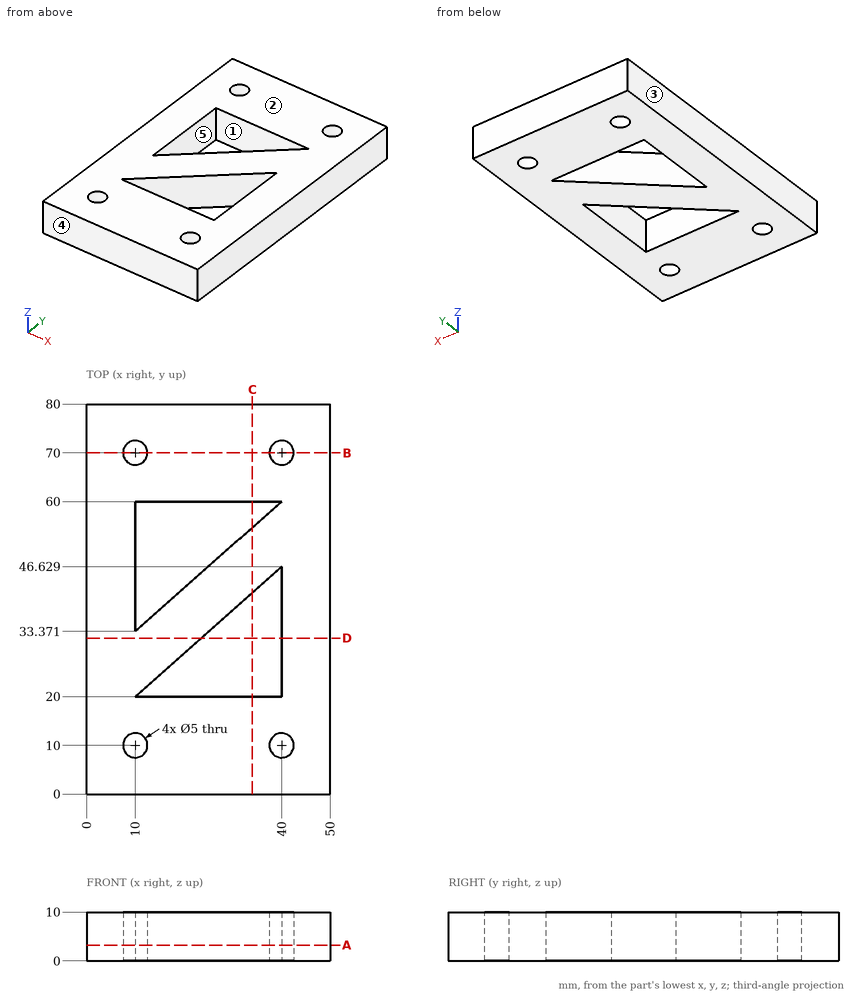
Geometry: see drawing. Coordinates: mm, zero at the bounding-box minimum. A direction names the side the tool comes from. Give positions to 0.01 mm unless a question says otherwise; leave off trailing zeros. Order: outer loops, then holes, each group sorted by start corner. A loop starts at its lowest first (then second) coordinate and runs counter-clockwise, first axis right, second up.
Q1. Section D-D on y = 32. Output: boundary loops of the cut face in (x, z), and give its area (3 significant figures).
Checked values:
outline: (0, 0) - (23.52, 0) - (23.52, 10) - (0, 10) - close; (40, 0) - (50, 0) - (50, 10) - (40, 10) - close
area: 335 mm2
Q2. Ray query, probe 1 along Y at (x, z) = (24, 8.5); probe 2 along Y at (x, z) = (33, 2.25) (1 decimal); probe 3 along X at (y, z) = (69.5, 8.75). Return the intervals inside material, ascending.
Checked values:
probe 1: y = 0 to 20, 32.43 to 45.8, 60 to 80
probe 2: y = 0 to 20, 40.4 to 53.8, 60 to 80
probe 3: x = 0 to 7.55, 12.45 to 37.55, 42.45 to 50
Q3. Contact query for a flat-ended pin moving along its axis: pin 1 Ø4 at (x, y) = (10, 10) entering from -Z. Output: stop coordinate, or through.
Checked values:
pin 1: passes through
Q4. Section B-B on y = 70. Output: boundary loops of the cut face in (x, z).
Checked values:
outline: (0, 0) - (7.5, 0) - (7.5, 10) - (0, 10) - close; (12.5, 0) - (37.5, 0) - (37.5, 10) - (12.5, 10) - close; (42.5, 0) - (50, 0) - (50, 10) - (42.5, 10) - close
Q5. Section C-C on x = 34. Output: boundary loops of the cut face in (y, z).
Checked values:
outline: (0, 0) - (20, 0) - (20, 10) - (0, 10) - close; (41.3, 0) - (54.67, 0) - (54.67, 10) - (41.3, 10) - close; (60, 0) - (80, 0) - (80, 10) - (60, 10) - close
Q6. Set-up query: the marked faces 1 and 2. Return all of +Z, -Z, +X, -X, +Y, -Y with unobstructed straight access to the full face (end or side cutting, diameter ignored); none if empty.
Checked values:
face 1: +Z, -Z
face 2: +Z, +X, -X, +Y, -Y
Q7. Draft query along Y for the marked faces 3, 4 and 5. Return one class per face: +Y half, -Y half, draft (parallel to the pull), parting line (faces both ways), or undercut.
Checked values:
face 3: draft
face 4: -Y half
face 5: undercut
Q8. Section A-A on z = 3.25. Output: boundary loops of the cut face in (x, y), and give its area (3 significant figures).
Checked values:
outline: (0, 0) - (50, 0) - (50, 80) - (0, 80) - close; hole circle Ø5 at (10, 10); hole circle Ø5 at (10, 70); hole (10, 20) - (40, 20) - (40, 46.63) - close; hole (10, 33.37) - (40, 60) - (10, 60) - close; hole circle Ø5 at (40, 10); hole circle Ø5 at (40, 70)
area: 3,120 mm2
